Part model, mm, in its own coordinate system. Face numbers are marked on the shaded views. A direction names the side the tool comes from. Give positions to 0.01 mm unless a question says otherwise; leave off trailing zeros. Order: outer loops, then holes, each group sorted by start corner. A loop starts at its lowest first (then second) coordinate and runs counter-clockwise, first axis right, second up. Notation, with made-up numbers: (38.25, 18) - (44.25, 18) arc R16 cw to (44.25, 46) - close; hole circle Ø11 at (79.25, 28). An arc over 180 degrees is marked (long way). One line per item, written item: value.
```python
from build123d import *

# Parameters (mm, degrees)
ESQUISSE3_W                  = 6.57785754
ESQUISSE3_H                  = 1.386048805
ENL_V_MAT_EXTRU_1_DEPTH      = 10.5
D_GAGEMENT_M21_D             = 2.4
R_P_TITION_CIRCULAIRE1_COUNT = 4
CONG_1_R                     = 0.05


with BuildPart() as part:
    # Esquisse2 → Révolution2 (revolve)
    with BuildSketch(Plane.XY, mode=Mode.PRIVATE) as r_volution2_sk:
        Polygon((0, 19), (3.15, 19), (3.15, 8.5), (6.2, 8.5), (6.2, 3), (6.2, 1), (10, 1), (10, 0), (0, 0), align=None)
    revolve(r_volution2_sk.sketch.rotate(Axis((0, 0, 0), (0, 1, 0)), 90), axis=Axis((0, 0, 0), (0, 1, 0)))

    # Esquisse3 → Enlèv. mat.-Extru.1 (cut)
    with BuildSketch(Plane(origin=(0, 19, 0), x_dir=(1, 0, 0), z_dir=(0, 1, 0))):
        with Locations((-0.352413472, 3.114928535)):
            Rectangle(ESQUISSE3_W, ESQUISSE3_H)
    extrude(amount=-ENL_V_MAT_EXTRU_1_DEPTH, mode=Mode.SUBTRACT)

    # Dégagement M21 (through all)
    with Locations(Plane(origin=(0, 1, 0), x_dir=(1, 0, 0), z_dir=(0, 1, 0))):
        with Locations((0.371303159, 7.991378727)):
            d_gagement_m21 = Hole(D_GAGEMENT_M21_D / 2)

    # Répétition circulaire1: Dégagement M21 ×4 about axis
    r_p_tition_circulaire1_axis = Axis((0, 0, 0), (0, 1, 0))
    for i in range(1, R_P_TITION_CIRCULAIRE1_COUNT):
        add(d_gagement_m21.rotate(r_p_tition_circulaire1_axis, i * 360 / R_P_TITION_CIRCULAIRE1_COUNT), mode=Mode.SUBTRACT)

    # Congé1
    cong_1_edges = [part.edges().sort_by_distance(p)[0] for p in [
        (0, 1, 6.2),
        (0, 8.5, 6.2),
        (0, 8.5, 3.15),
        (0, 19, 3.15),
    ]]
    fillet(cong_1_edges, radius=CONG_1_R)


solid = part.part
```
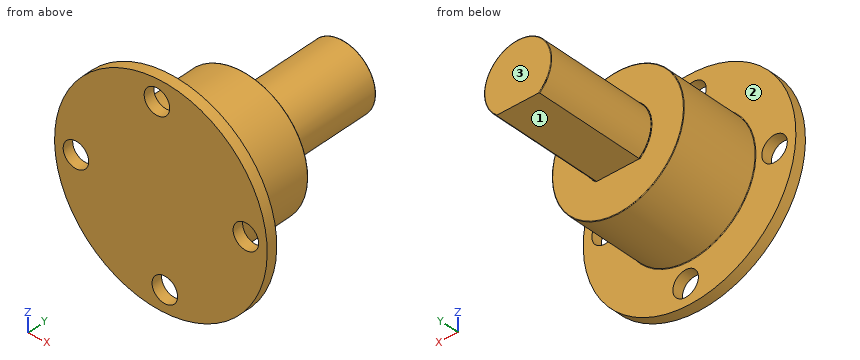
1) Slice it at B-B on z = 0. Write the cut outline in (x, y).
Answer:
outline: (-10, 0) - (-9.13, 0) - (-9.13, 1) - (-10, 1) - close; (-6.85, 0) - (6.85, 0) - (6.85, 1) - (6.25, 1) arc R0.05 cw to (6.2, 1.05) - (6.2, 8.45) arc R0.05 ccw to (6.15, 8.5) - (3.2, 8.5) arc R0.05 cw to (3.15, 8.55) - (3.15, 18.95) arc R0.05 ccw to (3.1, 19) - (-3.1, 19) arc R0.05 ccw to (-3.15, 18.95) - (-3.15, 8.55) arc R0.05 cw to (-3.2, 8.5) - (-6.15, 8.5) arc R0.05 ccw to (-6.2, 8.45) - (-6.2, 1.05) arc R0.05 cw to (-6.25, 1) - (-6.85, 1) - close; (9.13, 0) - (10, 0) - (10, 1) - (9.13, 1) - close
2) Drop flat-ended pins along their axis: P1, Ø2, axis at x = -3, z = -3.5, coming from the +Y side; P2, Ø2, axis at y = 15.5, z = 1.5, coming from the -X side; P3, Ø4, axis at x = -4.5, y = 9.5, coming from the +Z side. Give the stop position or say it passes through.
Answer:
P1: stops at y = 8.5
P2: stops at x = -3.11
P3: stops at z = 5.53
3) Slice it at A-A on x = 0. Write the cut outline in (y, z).
Answer:
outline: (0, -10) - (1, -10) - (1, -9.13) - (0, -9.13) - close; (0, -6.85) - (1, -6.85) - (1, -6.25) arc R0.05 cw to (1.05, -6.2) - (8.45, -6.2) arc R0.05 ccw to (8.5, -6.15) - (8.5, -2.42) - (19, -2.42) - (19, 3.1) arc R0.05 ccw to (18.95, 3.15) - (8.55, 3.15) arc R0.05 cw to (8.5, 3.2) - (8.5, 6.15) arc R0.05 ccw to (8.45, 6.2) - (1.05, 6.2) arc R0.05 cw to (1, 6.25) - (1, 6.85) - (0, 6.85) - close; (0, 9.13) - (1, 9.13) - (1, 10) - (0, 10) - close
4) Slice it at C-C on y = 9.75. Write the cut outline in (x, z), then the cut area to 3 significant figures.
Answer:
outline: (-2.01, -2.42) - (2.01, -2.42) arc R3.15 ccw (long way) to start
area: 29.2 mm2
5) Which spindle directions (+Z, -Z, +X, -X, +Y, -Y) get a long thin tool onto all of the face, cutting with end or side? Do the marked faces 1, 2 and 3. Say none if no direction does.
Answer:
face 1: -Z, +X, -X, +Y
face 2: +Y
face 3: +Z, -Z, +X, -X, +Y
6) Wall check: line 1 along Y through (x, z) = (-1.75, -4); line 2 along Y through (x, z) = (1, -6.5); line 3 along X through (y, z) = (1.25, -1.75). Give the ranges that are in metal, low to high. Write a range as [from, to].
Answer:
line 1: y = [0, 8.5]
line 2: y = [0, 1]
line 3: x = [-5.95, 5.95]
